```python
from build123d import *

# Parameters (mm, degrees)
F4_W     = 9.5127796691
F4_H     = 0.5
F4_W_2   = 0.5
F4_H_2   = 9.9936255533
F4_W_3   = 9.9872203309
F4_H_3   = 9.5063744467
F5_DEPTH = 25


with BuildPart() as f2:
    # F1 (on Front) → F2 (revolve)
    with BuildSketch(Plane.XZ):
        Polygon((0, 10), (-37.9932709038, 0), (0, 0), align=None)
    revolve(axis=Axis((0, 0, 0), (0, 0, 1)))

    # F4 (on offset) → F5 (cut)
    with BuildSketch(Plane.XY.offset(10.1)):
        with Locations((-4.9916676883, -0.0203696135)):
            Rectangle(F4_W, F4_H)
        with Locations((0.0147221462, 5.2264431631)):
            Rectangle(F4_W_2, F4_H_2)
        with Locations((0.0147221462, -0.0203696135)):
            Rectangle(F4_W_2, F4_H)
        with Locations((5.2583323117, -0.0203696135)):
            Rectangle(F4_W_3, F4_H)
        with Locations((0.0147221462, -5.0235568369)):
            Rectangle(F4_W_2, F4_H_3)
    extrude(amount=-F5_DEPTH, mode=Mode.SUBTRACT)


solid = f2.part
```
Build history of the part. All positions in model axes, mm. Give positions to 0.01 mm unless a question says otherwise; leave off trailing zeros. Loops run counter-clockwise (first coordinate to the right, second up) from the corner with the lowest first, then second, coordinate; pieces in that order, holes last. Notation, with made-up numbers: (-39, -35) -> (-27, -35) arc R5 cw to (-27, -28) -> close; hole circle Ø1 at (75.5, 65.5). An arc over 180 degrees is marked (long way). One line per question, with ' | ' between items. Start each with the question number.
1) Cut at A-A (z = 8.75). Give the cut face in (x, y), plus the area to 3 significant figures.
2) Two-plate mould, pull along Y, no slides. Class faces 1 (the flat face through (1, -1, 0)), 2 (the flat face through (0.265, 5, 4)), 3 (the conical face through (-2.561, -0.806, 9.293)), 4 (the flat face through (-5, 0.23, 4)): released by +Y, released by -Y, zero draft, split by the parting line, or undercut.
3) Pin check, flat tips, straight feed: pin 1 (4 mm diameter, centred on x = 0, y = -14.5, fed in from +Z); pin 2 (6 mm diameter, centred on x = 26, y = 16.5, fed in from +Z). Stop position of each tip, or through.
4) Cut at B-B (z = 2). Give the cut face in (x, y).
5) Probe L1, parallel to Z at x = 11, y = 35.5; L2, parallel to Z at x = 4, y = 25.5. List the from-to ranges inside material, lowest first.
Return value:
1) outline: (-4.74, -0.27) arc R4.75 ccw to (-0.24, -4.74) -> (-0.24, -0.27) -> close; (-4.74, 0.23) -> (-0.24, 0.23) -> (-0.24, 4.74) arc R4.75 ccw to start; (0.26, -4.74) arc R4.75 ccw to (4.74, -0.27) -> (0.26, -0.27) -> close; (0.26, 0.23) -> (4.74, 0.23) arc R4.75 ccw to (0.26, 4.74) -> close | area: 61.6 mm^2
2) face 1: zero draft | face 2: undercut | face 3: split by the parting line | face 4: undercut
3) pin 1: z = 6.71 | pin 2: z = 2.68
4) outline: circle Ø60.79 at (0, 0); hole (-9.75, -0.27) -> (-0.24, -0.27) -> (-0.24, -9.78) -> (0.26, -9.78) -> (0.26, -0.27) -> (10.25, -0.27) -> (10.25, 0.23) -> (0.26, 0.23) -> (0.26, 10.22) -> (-0.24, 10.22) -> (-0.24, 0.23) -> (-9.75, 0.23) -> close
5) L1: 0 to 0.22 | L2: 0 to 3.21
